Input: part model. Units: mm. Frame: model coordinates. Face numbers are marked on the shaded views. Round coordinates to 2 decimals unless told otherwise and drop trailing zeros. Loops run counter-clockwise (first coordinate to the right, second up) from the corner with the lowest first, then second, coordinate; pieces in that order, holes last.
(1) First-contact query: pin 1 Ø2 at (x, z) = (-5, 23.5) entering from +Y; pin 2 Ø6 at (x, z) = (-1.5, 6.5) entering from -Y; pin 3 Ø4 at (y, z) = (-2.5, 39.5) entering from -X; pin 4 Ø5 at (x, y) = (0, 0) entering from +Z. Flat tips, straight axial feed; report the tip coordinate or a pass-through.
(2) Draft query along X for the marked faces 1, 2 and 3. Return one class per face: released by +X, released by -X, zero draft, split by the parting line, or undercut.
(3) Line query: line 1 (Y direction, x = 0, z = 25.5) (3 decimals); line 2 (X direction, y = -2.75, z = 28); line 3 (X direction, y = -2.25, z = 48.5). Output: solid intervals per line, ascending.
(4) Cut plane C-C, the plane z = 19. Output: boundary loops of the cut face in (x, y) (3 decimals), and give its area (3 significant figures).
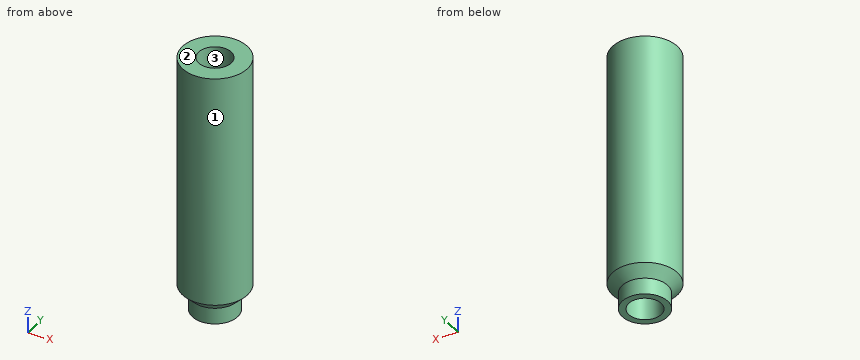
from build123d import *

# Parameters (mm, degrees)
SKETCH1_R           = 6.35
BOSS_EXTRUDE1_DEPTH = 50.8
SKETCH2_R           = 6.35
SKETCH2_R_2         = 4.445
CUT_EXTRUDE1_DEPTH  = 3.175
CHAMFER1_SIZE       = 1.905
SKETCH3_R           = 3.175
CUT_EXTRUDE2_DEPTH  = 52.587643869


with BuildPart() as part:
    # Sketch1 → Boss-Extrude1 (new body)
    with BuildSketch(Plane.XY):
        Circle(SKETCH1_R)
    extrude(amount=BOSS_EXTRUDE1_DEPTH)

    # Sketch2 → Cut-Extrude1 (cut)
    with BuildSketch(Plane(origin=(0, 0, 0), x_dir=(-1, 0, 0), z_dir=(0, 0, -1))):
        Circle(SKETCH2_R)
        Circle(SKETCH2_R_2, mode=Mode.SUBTRACT)
    extrude(amount=-CUT_EXTRUDE1_DEPTH, mode=Mode.SUBTRACT)

    # Chamfer1
    chamfer1_edges = [part.edges().sort_by_distance(p)[0] for p in [
        (-6.35, 0, 3.175),
    ]]
    chamfer(chamfer1_edges, length=CHAMFER1_SIZE - 0.0001)  # a hair under: the kernel refuses the full size

    # Sketch3 → Cut-Extrude2 (cut, through all)
    with BuildSketch(Plane(origin=(0, 0, 0), x_dir=(-1, 0, 0), z_dir=(0, 0, -1))):
        Circle(SKETCH3_R)
    extrude(amount=-CUT_EXTRUDE2_DEPTH, mode=Mode.SUBTRACT)


solid = part.part
Reported:
1. pin 1: stops at y = 4.93
1. pin 2: stops at y = -6.35
1. pin 3: stops at x = -6.33
1. pin 4: passes through
2. face 1: split by the parting line
2. face 2: zero draft
2. face 3: undercut
3. line 1: y = -6.35 to -3.175, 3.175 to 6.35
3. line 2: x = -5.72 to -1.59, 1.59 to 5.72
3. line 3: x = -5.94 to -2.24, 2.24 to 5.94
4. outline: circle Ø12.7 at (0, 0); hole circle Ø6.35 at (0, 0)
4. area: 95.0 mm2
